from build123d import *

# Parameters (mm, degrees)
F0_W      = 9.7
F0_H      = 7.1
F0_H_2    = 4.7
F0_W_2    = 2.5
F0_H_3    = 1.2
F1_DEPTH  = 25
F2_R      = 1
F3_R      = 2.1
F4_DEPTH  = 30
F6_DEPTH  = 8
F7_R      = 3.5
F8_DEPTH  = 5
F10_DEPTH = 6


with BuildPart() as f1:
    # F0 (on Top) → F1 (new body)
    with BuildSketch(Plane.XY):
        with Locations((-0.15, -0.179021287)):
            Rectangle(F0_W, F0_H)
        with Locations((-0.15, -6.079021287)):
            Rectangle(F0_W, F0_H_2)
        with Locations((-6.25, -6.079021287)):
            Rectangle(F0_W_2, F0_H_2)
        with Locations((5.95, -6.079021287)):
            Rectangle(F0_W_2, F0_H_2)
        with Locations((-0.15, -9.029021287)):
            Rectangle(F0_W, F0_H_3)
        Polygon((4.7, -9.629021287), (-5, -9.629021287), (0, -14.629021287), align=None)
    extrude(amount=F1_DEPTH)

    # F2
    f2_edges = [f1.edges().sort_by_distance(p)[0] for p in [
        (-7.5, -3.729021, 12.5),
        (-7.5, -8.429021, 12.5),
        (7.2, -3.729021, 12.5),
        (7.2, -8.429021, 12.5),
        (0, -14.629021, 12.5),
    ]]
    fillet(f2_edges, radius=F2_R)

    # F3 (on face) → F4 (cut)
    with BuildSketch(Plane(origin=(0, 3.370978713, 0), x_dir=(-1, 0, 0), z_dir=(0, 1, 0))):
        with Locations((0, 7.5)):
            Circle(F3_R)
        with Locations((0, 12)):
            Circle(F3_R)
        with Locations((0, 3)):
            Circle(F3_R)
        with Locations((0, 16.5)):
            Circle(F3_R)
    extrude(amount=-F4_DEPTH, mode=Mode.SUBTRACT)

    # F5 (on face) → F6 (join)
    with BuildSketch(Plane(origin=(0, 3.370978713, 0), x_dir=(-1, 0, 0), z_dir=(0, 1, 0))):
        with BuildLine():
            ThreePointArc((0, 25), (-1.3453995809, 24.4427172468), (-1.9026823342, 23.0973176658))
            ThreePointArc((-1.9026823342, 23.0973176658), (0, 21.1946353316), (1.9026823342, 23.0973176658))
            ThreePointArc((1.9026823342, 23.0973176658), (1.3453995809, 24.4427172468), (0, 25))
        make_face()
        with BuildLine():
            Line((-1.9026823342, 25), (-1.9026823342, 23.0973176658))
            ThreePointArc((-1.9026823342, 23.0973176658), (-1.3453995809, 24.4427172468), (0, 25))
            Line((0, 25), (-1.9026823342, 25))
        make_face()
        with BuildLine():
            ThreePointArc((0, 25), (1.3453995809, 24.4427172468), (1.9026823342, 23.0973176658))
            Line((1.9026823342, 23.0973176658), (1.9026823342, 25))
            Line((1.9026823342, 25), (0, 25))
        make_face()
    extrude(amount=F6_DEPTH)

    # F7 (on face) → F8 (cut)
    with BuildSketch(Plane.XY.offset(25)):
        with Locations((0, -1.629021287)):
            Circle(F7_R)
    extrude(amount=-F8_DEPTH, mode=Mode.SUBTRACT)

    # F9 (on face) → F10 (cut)
    with BuildSketch(Plane.YZ.offset(7.2)):
        with BuildLine():
            ThreePointArc((-6.079021287, 15.4), (-5.3012038277, 15.7221825407), (-4.979021287, 16.5))
            ThreePointArc((-4.979021287, 16.5), (-5.3012038277, 17.2778174593), (-6.079021287, 17.6))
            Line((-6.079021287, 17.6), (-6.079021287, 15.4))
        make_face()
        with BuildLine():
            ThreePointArc((-4.979021287, 3), (-5.3012038277, 3.7778174593), (-6.079021287, 4.1))
            Line((-6.079021287, 4.1), (-6.079021287, 1.9))
            ThreePointArc((-6.079021287, 1.9), (-5.3012038277, 2.2221825407), (-4.979021287, 3))
        make_face()
        with BuildLine():
            Line((-6.079021287, 1.9), (-6.079021287, 4.1))
            ThreePointArc((-6.079021287, 4.1), (-7.179021287, 3), (-6.079021287, 1.9))
        make_face()
        with BuildLine():
            ThreePointArc((-4.979021287, 7.5), (-5.3012038277, 8.2778174593), (-6.079021287, 8.6))
            Line((-6.079021287, 8.6), (-6.079021287, 6.4))
            ThreePointArc((-6.079021287, 6.4), (-5.3012038277, 6.7221825407), (-4.979021287, 7.5))
        make_face()
        with BuildLine():
            Line((-6.079021287, 6.4), (-6.079021287, 8.6))
            ThreePointArc((-6.079021287, 8.6), (-7.179021287, 7.5), (-6.079021287, 6.4))
        make_face()
        with BuildLine():
            ThreePointArc((-4.979021287, 12), (-5.3012038277, 12.7778174593), (-6.079021287, 13.1))
            Line((-6.079021287, 13.1), (-6.079021287, 10.9))
            ThreePointArc((-6.079021287, 10.9), (-5.3012038277, 11.2221825407), (-4.979021287, 12))
        make_face()
        with BuildLine():
            Line((-6.079021287, 10.9), (-6.079021287, 13.1))
            ThreePointArc((-6.079021287, 13.1), (-7.179021287, 12), (-6.079021287, 10.9))
        make_face()
        with BuildLine():
            Line((-6.079021287, 15.4), (-6.079021287, 17.6))
            ThreePointArc((-6.079021287, 17.6), (-7.179021287, 16.5), (-6.079021287, 15.4))
        make_face()
    extrude(amount=-F10_DEPTH, mode=Mode.SUBTRACT)


solid = f1.part
Design review of the part built by this model. Coordinates are the model's own, in mm. A direction names the side the tool comes from. Coordinates: 2 decimals unless noted, no trailing zeros. Loops run counter-clockwise (first coordinate to the right, second up) from the corner with the lowest first, then second, coordinate; pieces in that order, holes last. Notation, with made-up numbers: (14.5, 41.5) -> (63.5, 41.5) arc R14 ccw to (63.5, 68.5) -> close; hole circle Ø5 at (40, 76.5). An arc over 180 degrees is marked (long way). Use a Markdown table: item, result. Add a question column.
Item 1: The part is to be moulded in two halves that separate along Z. For faces 1 (the flat face through (5, -3.729, 12)), 2 (the cylindrical face through (-2.003, -5.288, 12.631)), 3 (the flat face through (0, -5, 0)), say which applies: +Z half, -Z half, draft (parallel to the pull), parting line (faces both ways), or undercut.
Item 2: We need section A-A, the plane x = 5.25. Write out the cut boundary in (y, z).
Item 3: Machinability: for faces 4 (the flat face through (1.903, 7, 24)), 5 (the flat face through (-6, -3.729, 12)), 6 (the flat face through (4.7, -9, 12)), which of the approach directions +Z, -Z, +X, -X, +Y, -Y give a long, thin tool a straight path to every point of the face, cutting with its end or side? Answer none if there is none.
Item 4: Wall thickness on L1, parallel to Z at x = 0, y = -6.5; L2, parallel to Z at x = 0, y = -1.75; L3, parallel to Y at x = 5, z = 18.25: over which ranges is each line inside the solid? List them lowest first. Write a range as from..to.
Item 5: We need section D-D, the plane x = -0.25. Write out the cut boundary in (y, z), and give its area (3 significant figures).
Item 6: We need section B-B, the plane y = -8.75. Write out the cut boundary in (x, z), and give its area (3 significant figures).
Item 7: Clearance check with flat-ended pins moving along their axes: P1, Ø6.5, axis at x = 0, z = 12, coming from the +Y side; P2, Ø0.6, axis at y = -9, z = 13, coming from the -X side; P3, Ø1, axis at x = -1.5, z = 16.5, coming from the +Y side; P4, Ø1.5, axis at y = 8.5, z = 24.5, coming from the +X side. State where each tip first meets the part, or that it passes through.
Item 8: We need section C-C, the plane z = 22. Write out the cut boundary in (x, y).
Numbers:
| question | item | result |
|---|---|---|
| 1 | face 1 | draft |
| 1 | face 2 | undercut |
| 1 | face 3 | -Z half |
| 2 | outline | (-8.43, 0) -> (-3.73, 0) -> (-3.73, 25) -> (-8.43, 25) -> close; hole circle Ø2.2 at (-6.08, 3); hole circle Ø2.2 at (-6.08, 7.5); hole circle Ø2.2 at (-6.08, 12); hole circle Ø2.2 at (-6.08, 16.5) |
| 3 | face 4 | +Z, -Z, +X, +Y |
| 3 | face 5 | +Z, -Z, -X, +Y |
| 3 | face 6 | +Z, -Z, +X, -Y |
| 4 | L1 | z = 0..0.9, 5.1..5.4, 9.6..9.9, 14.1..14.4, 18.6..25 |
| 4 | L2 | z = 0..0.9, 5.1..5.4, 9.6..9.9, 14.1..14.4, 18.6..20 |
| 4 | L3 | y = -8.43..-3.73 |
| 5 | outline | (-14.17, 0) -> (3.37, 0) -> (3.37, 0.91) -> (-14.17, 0.91) -> close; (-14.17, 5.09) -> (3.37, 5.09) -> (3.37, 5.41) -> (-14.17, 5.41) -> close; (-14.17, 9.59) -> (3.37, 9.59) -> (3.37, 9.91) -> (-14.17, 9.91) -> close; (-14.17, 14.09) -> (3.37, 14.09) -> (3.37, 14.41) -> (-14.17, 14.41) -> close; (-14.17, 18.59) -> (3.37, 18.59) -> (3.37, 21.21) -> (11.37, 21.21) -> (11.37, 25) -> (1.86, 25) -> (1.86, 20) -> (-5.12, 20) -> (-5.12, 25) -> (-14.17, 25) -> close |
| 5 | area | 141 mm^2 |
| 6 | outline | (-5, 0) -> (4.7, 0) -> (4.7, 25) -> (-5, 25) -> close; hole circle Ø4.2 at (0, 3); hole circle Ø4.2 at (0, 7.5); hole circle Ø4.2 at (0, 12); hole circle Ø4.2 at (0, 16.5) |
| 6 | area | 187 mm^2 |
| 7 | P1 | stops at y = 3.37 |
| 7 | P2 | stops at x = -5 |
| 7 | P3 | passes through |
| 7 | P4 | stops at x = 1.9 |
| 8 | outline | (-7.5, -7.43) arc R1 ccw to (-6.5, -8.43) -> (-5, -8.43) -> (-5, -9.63) -> (-0.73, -13.9) arc R1 ccw to (0.71, -13.88) -> (4.7, -9.63) -> (4.7, -8.43) -> (6.2, -8.43) arc R1 ccw to (7.2, -7.43) -> (7.2, -4.73) arc R1 ccw to (6.2, -3.73) -> (4.7, -3.73) -> (4.7, 3.37) -> (1.55, 3.37) -> (1.55, 11.37) -> (-1.55, 11.37) -> (-1.55, 3.37) -> (-5, 3.37) -> (-5, -3.73) -> (-6.5, -3.73) arc R1 ccw to (-7.5, -4.73) -> close; hole circle Ø7 at (0, -1.63) |
